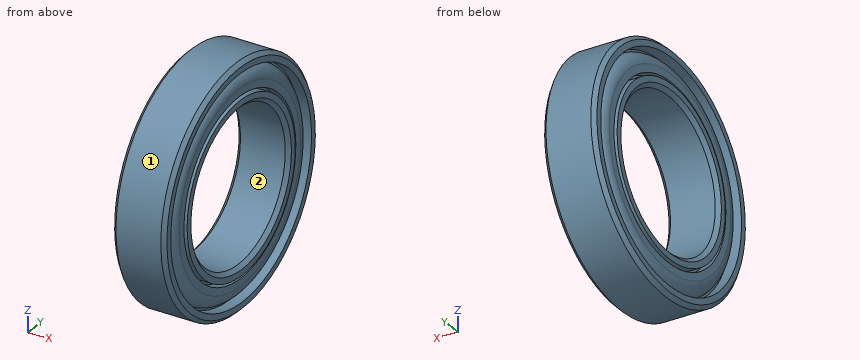
```python
from build123d import *

# Parameters (mm, degrees)
SKETCH2_W     = 7
SKETCH2_H     = 6
FILLET1_R     = 1.8
CHAMFER1_SIZE = 0.5


with BuildPart() as part:
    # Sketch2 → Revolve1 (revolve)
    with BuildSketch(Plane.XY, mode=Mode.PRIVATE) as revolve1_sk:
        with Locations((0, 13)):
            Rectangle(SKETCH2_W, SKETCH2_H)
    revolve(revolve1_sk.sketch.rotate(Axis((0, 0, 0), (-1, 0, 0)), 90), axis=Axis((0, 0, 0), (-1, 0, 0)))

    # Sketch4 → Cut-Revolve1 (revolve, cut)
    with BuildSketch(Plane.XY, mode=Mode.PRIVATE) as cut_revolve1_sk:
        Polygon((6.594167107, 14.707924858), (2.022867053, 14.707924858), (2.022867053, 14.424029148), (3.332429366, 14.424029148), (3.332429366, 11.692719364), (2.022867053, 11.692719364), (2.022867053, 11.291318583), (6.594167107, 11.291318583), align=None)
        Polygon((-6.594167107, 11.291318583), (-6.594167107, 14.707924858), (-2.022867053, 14.707924858), (-2.022867053, 14.424029148), (-3.332429366, 14.424029148), (-3.332429366, 11.692719364), (-2.022867053, 11.692719364), (-2.022867053, 11.291318583), align=None)
    revolve(cut_revolve1_sk.sketch.rotate(Axis((0, 0, 0), (1, 0, 0)), 90), axis=Axis((0, 0, 0), (1, 0, 0)), mode=Mode.SUBTRACT)

    # Fillet1
    # the kernel refuses this fillet: 1.8 mm, written as the material it takes off along each edge
    with BuildSketch(Plane(origin=(3.332429366, 0, 0), x_dir=(0, 0, 1), z_dir=(0, 1, 0))) as fillet1_piece_1:
        with BuildLine():
            CenterArc((12.692131092, -1.8), FILLET1_R, 15.811024237, 74.188975763)
            Line((12.692131092, 0), (12.692131092, 0.036))
            Line((12.692131092, 0.036), (14.424029148, 0.036))
            Line((14.424029148, 0.036), (14.460029148, 0))
            ThreePointArc((14.460029148, 0), (14.460029148, -0.654781157), (14.458667109, -1.299753559))
            Line((14.458667109, -1.299753559), (14.424029148, -1.309562313))
        make_face()
    revolve(axis=Axis((3.332429366, 0, 0), (1, 0, 0)), mode=Mode.SUBTRACT)
    with BuildSketch(Plane(origin=(-3.332429366, 0, 0), x_dir=(0, 0, 1), z_dir=(0, 1, 0))) as fillet1_piece_2:
        with BuildLine():
            CenterArc((12.692131092, 1.8), FILLET1_R, 270, 74.188975763)
            Line((12.692131092, 0), (12.692131092, -0.036))
            Line((12.692131092, -0.036), (14.424029148, -0.036))
            Line((14.424029148, -0.036), (14.460029148, 0))
            ThreePointArc((14.460029148, 0), (14.460029148, 0.654781157), (14.458667109, 1.299753559))
            Line((14.458667109, 1.299753559), (14.424029148, 1.309562313))
        make_face()
    revolve(axis=Axis((-3.332429366, 0, 0), (1, 0, 0)), mode=Mode.SUBTRACT)

    # Chamfer1
    chamfer1_edges = [part.edges().sort_by_distance(p)[0] for p in [
        (3.5, 0, 10),
        (-3.5, 0, 10),
        (-3.5, 0, 16),
        (3.5, 0, 16),
    ]]
    chamfer(chamfer1_edges, length=CHAMFER1_SIZE)


solid = part.part
```
Model file for the job. Use its own axes, mm. Face numbers are marked on the shaded views. Give positions to 0.01 mm unless a question says otherwise; leave off trailing zeros. Loops run counter-clockwise (first coordinate to the right, second up) from the corner with the lowest first, then second, coordinate; pieces in that order, holes last. Notation, with made-up numbers: (24.5, 40.25) -> (79.5, 40.25) arc R16 cw to (79.5, 57.25) -> close; hole circle Ø6 at (41.5, 17.5). An arc over 180 degrees is marked (long way). Use CSV: the item, a comma, the result in double quotes. Start each with the question number.
1) Slice it at A-A on x = -2.5. Give the cut face in (y, z).
2) Flat gauge pins, fed straight in: pin 1 Ø3 at (x, z) = (-1, 11) entering from +Y; pin 2 Ø1.5 at (x, y) = (-2.5, 11) entering from -Z; pin 3 Ø3 at (x, z) = (-1.5, 6) entering from -Y. Where does each tip first touch, or does it go through?
3) Wall check: line 1 (Y direction, x = 2.8, z = 0); line 2 (Y direction, x = -1.5, z = 0); line 3 (Z direction, x = 2.25, y = -3). Give the ranges that are in metal, low to high.
4) Mould opens along Y. For the marked faces 1 and 2 say: released by +Y, released by -Y, zero draft, split by the parting line, or undercut.
5) Slice it at B-B on x = -0.5. Give the cut face in (y, z).
Computed values:
1,outline,"circle Ø32 at (0, 0); circle Ø28.42 at (0, 0); circle Ø22.58 at (0, 0); hole circle Ø29.42 at (0, 0); hole circle Ø23.39 at (0, 0); hole circle Ø20 at (0, 0)"
2,pin 1,"stops at y = 12.87"
2,pin 2,"stops at z = -12.29"
2,pin 3,"stops at y = -15.35"
3,line 1,"y = -16 to -14.71, -13.97 to -11.69, -11.29 to -10, 10 to 11.29, 11.69 to 13.97, 14.71 to 16"
3,line 2,"y = -16 to -10, 10 to 16"
3,line 3,"z = -15.72 to -14.4, -14.03 to -11.3, -10.89 to -9.54, 9.54 to 10.89, 11.3 to 14.03, 14.4 to 15.72"
4,face 1,"split by the parting line"
4,face 2,"undercut"
5,outline,"circle Ø32 at (0, 0); hole circle Ø20 at (0, 0)"
